Model file for the job. Use its own axes, mm. A direction names the side the tool comes from. Round coordinates to 2 decimals unless told otherwise and drop trailing zeros. Order: outer loops, then holes, each group sorted by start corner. A loop starts at its lowest first (then second) coordinate and runs counter-clockwise, first axis right, second up. Notation, with made-up numbers: (62.5, 60.25) -> (109.5, 60.25) arc R21 cw to (109.5, 83.25) -> close; hole circle Ø2 at (47.25, 67). An arc over 180 degrees is marked (long way). Put each result on its own line as item: value. Start each with the question number.
Q1. 3-axis set-ups, long thin cutter, end or side, ignore diameter. For faces 5 (the face through (28.411, 4, 32)), 6 (the face through (-1, 45.183, 18)), 7 (the face through (-8, 29, 37.084)): which of +Z, -Z, +X, -X, +Y, -Y reach the whole face in a straight line?
Q2. Cut at C-C, the plane y = -9.5. List the corners of the cut face in (x, z).
Q3. Cut at D-D, the plane z = 38.5. List the corners of the cut face in (x, y), and give its area (3 significant figures).
Q4. Cut at B-B, the plane x = -36. List the corners of the cut face in (y, z).
Q5. Probe L1, parallel to Z at x = 0, y = 34; L2, parallel to X at y = 5, z = 34; L3, parallel to Z at x = -11, y = 42. List the from-to ranges inside material, lowest first.
Q6. Flat gauge pins, fed straight in: P1, Ø4, axis at x = 2, y = 2.5, coming from the +Z side; P2, Ø16.5, axis at x = 9, z = 9, coming from the -Y side. Where does each tip first touch, or does it go through?
Q7. Cut at A-A, the plane y = 39. List the corners of the cut face in (x, z), and give its area (3 significant figures).
Q8. Pull direction Z, two halves, no side cores. Call faces 1 (the face through (-7, -14.369, 7)), 2 (the face through (0.981, 19.078, 5.754)), 3 (the face through (-1, 10, 0)), 4 (the face through (36, 29, 47.498)): released by +Z, released by -Z, zero draft, split by the parting line, or undercut.
from build123d import *

# Parameters (mm, degrees)
F0_W        = 72.4030919373
F0_H        = 90.3663933277
F2_DEPTH    = 22.098
F1_W        = 15.5804120004
F1_H        = 90.3663933277
F3_DEPTH    = 32.512
F4_T1_DEPTH = 219.7018507435
F5_T1_DEPTH = 310.1779296127
F6_R        = 4.5271504528
F7_DEPTH    = 71.9636861302
F8_DEPTH    = 14.986


# Not quite as in the source:
# - a fillet or chamfer that OpenCascade refuses, or shapes differently, is made with other operations: its cross-section is extruded or revolved along the edge and cut away or added


with BuildPart() as f2:
    # F0 (on Top) → F2 (new body)
    with BuildSketch(Plane.XY):
        with Locations((-7.7902060002, 0)):
            Rectangle(F0_W, F0_H)
    extrude(amount=F2_DEPTH)

    # F1 (on face) → F3 (join)
    with BuildSketch(Plane.XY):
        with Locations((36.2015459687, 0)):
            Rectangle(F1_W, F1_H)
    extrude(amount=F3_DEPTH)

    # F4: chamfer of 57.15 x 47.9545439218 on 1 edges, made by hand

    # F4_s2 → F4_t1 (cut)
    with BuildSketch(Plane.YZ.offset(-191.290510775)):
        Polygon((11.9668033361, 22.098), (-45.1831966639, -25.8565439218), (-45.1831966639, 22.098), align=None)
    extrude(amount=F4_T1_DEPTH, mode=Mode.SUBTRACT)

    # F5: chamfer of 57.15 x 47.9545439218 on 1 edges, made by hand

    # F5_s2 → F5_t1 (cut)
    with BuildSketch(Plane.YZ.offset(-118.8874188377)):
        Polygon((11.9668033361, 32.512), (-45.1831966639, -15.4425439218), (-45.1831966639, 32.512), align=None)
    extrude(amount=F5_T1_DEPTH, mode=Mode.SUBTRACT)

    # F6 (on face) → F7 (cut, through all)
    with BuildSketch(Plane(origin=(0, 45.1831966639, 0), x_dir=(-1, 0, 0), z_dir=(0, 1, 0))):
        with Locations((0, 10.1730925962)):
            Circle(F6_R)
    extrude(amount=-F7_DEPTH, mode=Mode.SUBTRACT)

    # F8 (add): faces of the model
    f8_faces = [f2.faces().sort_by_distance(p)[0] for p in [
        (-7.7902060002, 28.575, 22.098),
        (-8.1168519447, -1.1571124664, 11.0857270906),
        (36.2015459687, -7.4063430651, 16.256),
        (36.2015459687, 28.575, 32.512),
    ]]
    extrude(f8_faces, amount=F8_DEPTH, dir=(0, 0, 1))


solid = f2.part
Ans:
1. face 5: +Z, -X, -Y
1. face 6: +Z, -Z, +X, -X, +Y
1. face 7: +Z, -X, +Y, -Y
2. outline: (-43.99, 0) -> (43.99, 0) -> (43.99, 29.49) -> (28.41, 29.49) -> (28.41, 19.07) -> (-43.99, 19.07) -> close
3. outline: (28.41, 1.24) -> (43.99, 1.24) -> (43.99, 45.18) -> (28.41, 45.18) -> close
3. area: 685 mm^2
4. outline: (-14.37, 0) -> (45.18, 0) -> (45.18, 37.08) -> (11.97, 37.08) -> (-14.37, 14.99) -> close
5. L1: z = 0 to 5.65, 14.7 to 37.08
5. L2: x = 28.41 to 43.99
5. L3: z = 0 to 37.08
6. P1: stops at z = 30.82
6. P2: stops at y = -14.37
7. outline: (-43.99, 0) -> (43.99, 0) -> (43.99, 47.5) -> (28.41, 47.5) -> (28.41, 37.08) -> (-43.99, 37.08) -> close; hole circle Ø9.05 at (0, 10.17)
7. area: 3,360 mm^2
8. face 1: zero draft
8. face 2: undercut
8. face 3: released by -Z
8. face 4: released by +Z
